Source: CAD feature listing. Evaluate the final solid. Frame: model axes, mm. A direction names the side the tool comes from. Round coordinates to 2 decimals unless told otherwise and drop trailing zeros. Order: outer loops, then holes, each group sorted by start corner. A loop starts at its lowest first (then second) coordinate and runs counter-clockwise, first axis right, second up. Notation, with made-up numbers: (-29.75, -26) -> (-16.75, -26) arc R21 cw to (-16.75, -16) -> close; hole circle Ø1 at (89.5, 21.5). An arc over 180 degrees is marked (long way). Write item = value, one per line. Start each with the question number.
(1) Cut plane B-B on x = 0. Return the cut outline in (y, z), then the cut area to 3 significant figures.
(2) Contact query for flat-ended pins moving along their axis: pin 1 Ø3 at (x, y) = (-0.5, -7) entering from +Z; pin 2 Ø5 at (x, y) = (0, -3) entering from -Z; pin 3 Ø3.5 at (y, z) = (-5, -0.5) entering from +X. Output: stop coordinate, or through.
(3) Cut plane C-C on y = 0.25. Return the cut outline in (x, z).
(4) Cut plane A-A on y = -1.75. Return the cut outline in (x, z).
(5) Cut plane D-D on y = -5.5. Return the cut outline in (x, z), then the cut area to 3 significant figures.
(6) Reachability of faces 1 (the face through (-6.3, -5, 0)), 2 (the face through (0, -2, -0.25)), 3 (the face through (-5.8, -4.9, -2)) from +Z, -Z, +X, -X, +Y, -Y: full face, straight path, thin tool, end or side. Return the list, or none.
(7) Ray query, line 1 (Z direction, x = 2.5, y = -4); line 2 (X direction, y = -3.5, z = -0.75); line 3 (Z direction, x = -2.75, y = 0.25). Return the intervals inside material, ascending.
(8) Draft query along Z for faces 4 (the face through (6.238, 1.329, -2.387)), 5 (the face through (-4.2, -2, 0)), 6 (the face through (6.697, 0.296, 2.959)). Return one class per face: released by +Z, released by -Z, zero draft, split by the parting line, or undercut.
from build123d import *

# Parameters (mm, degrees)
BOSS_EXTRUDE1_DEPTH = 1.6
CHAMFER1_SIZE       = 1
SKETCH3_W           = 12.6
SKETCH3_H           = 5
BOSS_EXTRUDE2_DEPTH = 11
CHAMFER2_SIZE       = 1
CUT_EXTRUDE1_DEPTH  = 6.65
SKETCH4_W           = 6
SKETCH4_H           = 0.5
BOSS_EXTRUDE3_DEPTH = 6


with BuildPart() as part:
    # Sketch1 → Boss-Extrude1 (new body)
    with BuildSketch(Plane(origin=(0, 0, 0), x_dir=(1, 0, 0), z_dir=(0, 1, 0))):
        with BuildLine():
            Line((-3.9, -4.1), (3.9, -4.1))
            ThreePointArc((3.9, -4.1), (6.728427125, -2.928427125), (7.9, -0.1))
            Line((7.9, -0.1), (7.9, 0.1))
            ThreePointArc((7.9, 0.1), (6.728427125, 2.928427125), (3.9, 4.1))
            Line((3.9, 4.1), (-3.9, 4.1))
            ThreePointArc((-3.9, 4.1), (-6.728427125, 2.928427125), (-7.9, 0.1))
            Line((-7.9, 0.1), (-7.9, -0.1))
            ThreePointArc((-7.9, -0.1), (-6.728427125, -2.928427125), (-3.9, -4.1))
        make_face()
    extrude(amount=BOSS_EXTRUDE1_DEPTH)

    # Chamfer1
    chamfer1_edges = [part.edges().sort_by_distance(p)[0] for p in [
        (6.728427125, 1.6, -2.928427125),
        (0, 1.6, -4.1),
        (-6.728427125, 1.6, -2.928427125),
        (-7.9, 1.6, 0),
        (-6.728427125, 1.6, 2.928427125),
        (0, 1.6, 4.1),
        (6.728427125, 1.6, 2.928427125),
        (7.9, 1.6, 0),
    ]]
    chamfer(chamfer1_edges, length=CHAMFER1_SIZE)

    # Sketch3 → Boss-Extrude2 (add)
    with BuildSketch(Plane.XZ):
        Rectangle(SKETCH3_W, SKETCH3_H)
    extrude(amount=BOSS_EXTRUDE2_DEPTH)

    # Chamfer2
    chamfer2_edges = [part.edges().sort_by_distance(p)[0] for p in [
        (-6.3, -5.5, 2.5),
        (-6.3, -5.5, -2.5),
        (6.3, -5.5, -2.5),
        (6.3, -5.5, 2.5),
        (-6.3, -11, 0),
        (0, -11, -2.5),
        (6.3, -11, 0),
        (0, -11, 2.5),
    ]]
    chamfer(chamfer2_edges, length=CHAMFER2_SIZE)

    # Sketch2 → Cut-Extrude1 (cut)
    with BuildSketch(Plane(origin=(0, 1.6, 0), x_dir=(1, 0, 0), z_dir=(0, 1, 0))):
        with BuildLine():
            Line((-3.7, -1.3), (3.7, -1.3))
            ThreePointArc((3.7, -1.3), (4.053553391, -1.153553391), (4.2, -0.8))
            Line((4.2, -0.8), (4.2, 0.8))
            ThreePointArc((4.2, 0.8), (4.053553391, 1.153553391), (3.7, 1.3))
            Line((3.7, 1.3), (-3.7, 1.3))
            ThreePointArc((-3.7, 1.3), (-4.053553391, 1.153553391), (-4.2, 0.8))
            Line((-4.2, 0.8), (-4.2, -0.8))
            ThreePointArc((-4.2, -0.8), (-4.053553391, -1.153553391), (-3.7, -1.3))
        make_face()
    extrude(amount=-CUT_EXTRUDE1_DEPTH, mode=Mode.SUBTRACT)

    # Sketch4 → Boss-Extrude3 (add)
    with BuildSketch(Plane(origin=(0, -5.05, 0), x_dir=(1, 0, 0), z_dir=(0, 1, 0))):
        Rectangle(SKETCH4_W, SKETCH4_H)
    extrude(amount=BOSS_EXTRUDE3_DEPTH)


solid = part.part
Evaluation:
q1.outline = (-11, -1.5) -> (-10, -2.5) -> (0, -2.5) -> (0, -4.1) -> (0.6, -4.1) -> (1.6, -3.1) -> (1.6, -1.3) -> (-5.05, -1.3) -> (-5.05, -0.25) -> (0.95, -0.25) -> (0.95, 0.25) -> (-5.05, 0.25) -> (-5.05, 1.3) -> (1.6, 1.3) -> (1.6, 3.1) -> (0.6, 4.1) -> (0, 4.1) -> (0, 2.5) -> (-10, 2.5) -> (-11, 1.5) -> close
q1.area = 51.8 mm^2
q2.pin_1 = 2.5
q2.pin_2 = -2.5
q2.pin_3 = 6.3
q3.outline = (-7.9, -0.1) arc R4 ccw to (-3.9, -4.1) -> (3.9, -4.1) arc R4 ccw to (7.9, -0.1) -> (7.9, 0.1) arc R4 ccw to (3.9, 4.1) -> (-3.9, 4.1) arc R4 ccw to (-7.9, 0.1) -> close; (-3, -0.25) -> (3, -0.25) -> (3, 0.25) -> (-3, 0.25) -> close; hole (-4.2, -0.8) arc R0.5 ccw to (-3.7, -1.3) -> (3.7, -1.3) arc R0.5 ccw to (4.2, -0.8) -> (4.2, 0.8) arc R0.5 ccw to (3.7, 1.3) -> (-3.7, 1.3) arc R0.5 ccw to (-4.2, 0.8) -> close
q4.outline = (-6.3, -1.5) -> (-5.3, -2.5) -> (5.3, -2.5) -> (6.3, -1.5) -> (6.3, 1.5) -> (5.3, 2.5) -> (-5.3, 2.5) -> (-6.3, 1.5) -> close; (-3, -0.25) -> (3, -0.25) -> (3, 0.25) -> (-3, 0.25) -> close; hole (-4.2, -0.8) arc R0.5 ccw to (-3.7, -1.3) -> (3.7, -1.3) arc R0.5 ccw to (4.2, -0.8) -> (4.2, 0.8) arc R0.5 ccw to (3.7, 1.3) -> (-3.7, 1.3) arc R0.5 ccw to (-4.2, 0.8) -> close
q5.outline = (-6.3, -1.5) -> (-5.3, -2.5) -> (5.3, -2.5) -> (6.3, -1.5) -> (6.3, 1.5) -> (5.3, 2.5) -> (-5.3, 2.5) -> (-6.3, 1.5) -> close
q5.area = 61.0 mm^2
q6.face_1 = +Z, -Z, -X, -Y
q6.face_2 = +Y
q6.face_3 = -Z, -X, -Y
q7.line_1 = -2.5 to -1.3, -0.25 to 0.25, 1.3 to 2.5
q7.line_2 = -6.3 to -4.2, 4.2 to 6.3
q7.line_3 = -4.1 to -1.3, -0.25 to 0.25, 1.3 to 4.1
q8.face_4 = released by -Z
q8.face_5 = undercut
q8.face_6 = released by +Z
